```python
from build123d import *

# Parameters (mm, degrees)
BOSS_EXTRUDE1_DEPTH     = 40
SKETCH6_R               = 1.5
CUT_EXTRUDE4_DEPTH      = 6.656854249
CUT_EXTRUDE4_DEPTH_BACK = 36.638181772
SKETCH9_R               = 1.5
CUT_EXTRUDE5_DEPTH      = 6.65685432
CUT_EXTRUDE5_DEPTH_BACK = 36.638181913
SKETCH16_R              = 1.5
CUT_EXTRUDE8_DEPTH      = 10
CUT_EXTRUDE8_DEPTH_BACK = 2.5


with BuildPart() as part:
    # Sketch2 → Boss-Extrude1 (new body)
    with BuildSketch(Plane.XY):
        with BuildLine():
            Line((10, 12.44732577), (0, 12.44732577))
            Line((0, 12.44732577), (0, 5.594433175))
            Line((0, 5.594433175), (0, 1.44732577))
            ThreePointArc((0, 1.44732577), (6.08276253, -0.615420297), (9.656086164, -5.95267423))
            Line((9.656086164, -5.95267423), (10, -5.95267423))
            Line((10, -5.95267423), (10, 12.44732577))
        make_face()
        with BuildLine():
            Line((0, 5.594433175), (0, 12.44732577))
            Line((0, 12.44732577), (-10, 12.44732577))
            Line((-10, 12.44732577), (-10, -5.95267423))
            Line((-10, -5.95267423), (-9.656086164, -5.95267423))
            ThreePointArc((-9.656086164, -5.95267423), (-6.08276253, -0.615420297), (0, 1.44732577))
            Line((0, 1.44732577), (0, 5.594433175))
        make_face()
    extrude(amount=BOSS_EXTRUDE1_DEPTH)

    # Sketch6 → Cut-Extrude4 (cut, two sides)
    with BuildSketch(Plane(origin=(0, 22.223662885, 22.223662885), x_dir=(0, -0.707106781, 0.707106781), z_dir=(0, 0.707106781, 0.707106781))) as cut_extrude4_sk:
        with Locations((25.139537037, 0)):
            Circle(SKETCH6_R)
    extrude(amount=CUT_EXTRUDE4_DEPTH, mode=Mode.SUBTRACT)
    extrude(cut_extrude4_sk.sketch, amount=-CUT_EXTRUDE4_DEPTH_BACK, mode=Mode.SUBTRACT)

    # Sketch9 → Cut-Extrude5 (cut, two sides)
    with BuildSketch(Plane(origin=(0, 2.223662885, -2.223662885), x_dir=(0, 0.707106781, 0.707106781), z_dir=(0, 0.707106781, -0.707106781))) as cut_extrude5_sk:
        with Locations((3.14473421, 0)):
            Circle(SKETCH9_R)
    extrude(amount=CUT_EXTRUDE5_DEPTH, mode=Mode.SUBTRACT)
    extrude(cut_extrude5_sk.sketch, amount=-CUT_EXTRUDE5_DEPTH_BACK, mode=Mode.SUBTRACT)

    # Sketch16 → Cut-Extrude8 (cut, two sides)
    with BuildSketch(Plane.XZ.offset(-1.44732577)) as cut_extrude8_sk:
        with Locations((0, 20)):
            Circle(SKETCH16_R)
    extrude(amount=CUT_EXTRUDE8_DEPTH, mode=Mode.SUBTRACT)
    extrude(cut_extrude8_sk.sketch, amount=-CUT_EXTRUDE8_DEPTH_BACK, mode=Mode.SUBTRACT)


solid = part.part
```
Design review of the part built by this model. Coordinates are the model's own, in mm. Give positions to 0.01 mm unless a question says otherwise; leave off trailing zeros. Loops run counter-clockwise (first coordinate to the right, second up) from the corner with the lowest first, then second, coordinate; pieces in that order, holes last. Notation, with made-up numbers: M -22,19 L 22,19 A32 ccw 22,58 Z; hole C -10,31 d4. An arc over 180 degrees is marked long. Return JSON: item names as keys, results as strings. Group by question number.
Item 1: We need section A-A (y = -0.5). Give the boundary of the cut face in (x, z), and give its area (3 significant figures).
Item 2: For probe 1 along X at (y, z) = (2.15, 20); probe 2 along Y at (x, z) = (-1.5, 16.5); probe 3 along Y at (x, z) = (2.75, 2), list the stretches that pass through material, from the lowest coordinate up.
Item 3: We need section C-C (x = 7.25). Give the boundary of the cut face in (y, z), and give its area (4 significant figures).
Item 4: We need section B-B (z = 32.5). Give the boundary of the cut face in (x, y), and give its area (3 significant figures).
Item 5: We need section D-D (x = -5.5). Give the boundary of the cut face in (y, z), and give its area (3 significant figures).
Item 6: Insertion check: pin 1 Ø3.5 at (x, z) = (0.5, 20.5) entering from -Y. The pin has a flat end and moves straight along its axis. Give the tip position at first contact, or say it passes through.
Item 7: Mouldability with a two-part tool opening along Z and no side actions: class faces 1 (the flat face through (0, 7, 0)), 2 (the flat face through (0, 12.447, 20)), 3 (the cylindrical face through (0.066, 3.971, 37.405)), 4 (the flat face through (0, 3.947, 20)) as released by +Z, released by -Z, zero draft, split by the parting line, or undercut.
Output:
{
 "1": {"outline": "M -10,0 L -5.93,0 L -5.93,40 L -10,40 Z; M 5.93,0 L 10,0 L 10,40 L 5.93,40 Z", "area": "326 mm^2"},
 "2": {"probe 1": "x = -10 to -1.5, 1.5 to 10", "probe 2": "y = 1.33 to 12.45", "probe 3": "y = 1.06 to 12.45"},
 "3": {"outline": "M -1.67,0 L 12.45,0 L 12.45,40 L -1.67,40 Z", "area": "564.5 mm^2"},
 "4": {"outline": "M -10,-5.95 L -9.66,-5.95 A10 cw 9.66,-5.95 L 10,-5.95 L 10,12.45 L -10,12.45 Z", "area": "262 mm^2"},
 "5": {"outline": "M -0.2,0 L 12.45,0 L 12.45,40 L -0.2,40 Z", "area": "506 mm^2"},
 "6": {"pin 1": "stops at y = 1.19"},
 "7": {"face 1": "released by -Z", "face 2": "zero draft", "face 3": "undercut", "face 4": "undercut"}
}
